Study the drawing (mm; zero at the part's minimum x, y, z) and answer. Round coordinates to 2 decimals unless told otherwise and drop trailing zeros. Order: outer loops, then holes, each group sorted by start corner. A loop starts at its lowest first (then second) coordinate and runs counter-clockwise, first axis right, second up. Notation, with made-up numbers: M 40.25,31 L 81.25,31 A5 ccw 81.25,40 Z; hole C 43.25,64.5 d11. An arc over 180 degrees is marked long. Put each result on its own line as item: value. Start each with the question number.
1. Each of these flat-tipped pins is pushed along its axis until it touches: pin 1 Ø2 at (y, z) = (470.5, 16) entering from -X; pin 2 Ø4 at (y, z) = (158.5, 12) entering from +X. Where does it stop, or does it pass through?
2. Consider line 1 (X direction, y = 190.5, z = 8.5); line 2 (X direction, y = 394.5, z = 9). Determine where each line is inside the solid, lowest interval first.
3. The part is cut by section B-B (z = 8.25). Give the vertices of the cut face in (x, y), then the cut area to 3 significant figures.
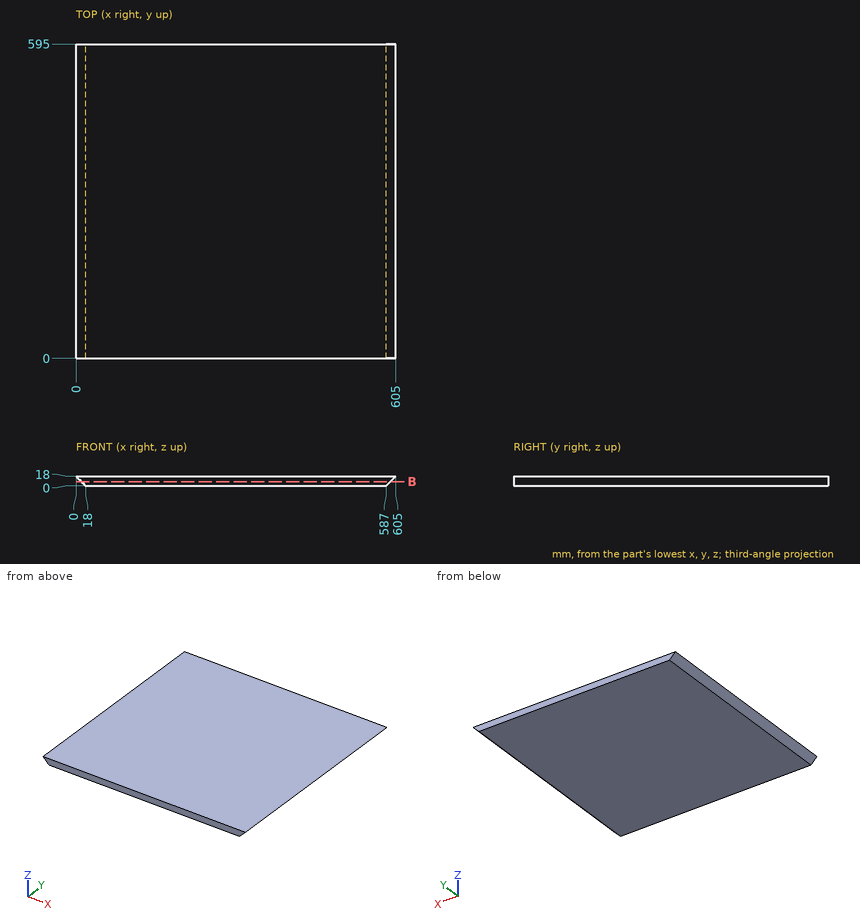
Resolved:
1. pin 1: x = 1
1. pin 2: x = 601
2. line 1: 9.5 to 595.5
2. line 2: 9 to 596
3. outline: M 9.75,0 L 595.25,0 L 595.25,595 L 9.75,595 Z
3. area: 348,000 mm2
